from build123d import *

# Parameters (mm, degrees)
EXTRUDE_1_DEPTH          = 64
CUT_EXTRUDE_1_DEPTH      = 850.57468483
CUT_EXTRUDE_1_DEPTH_BACK = 850.57468483
SKETCH_2_R               = 20
SKETCH_4_R               = 140
EXTRUDE_4_DEPTH          = 500
SHELL_6_T                = -5


with BuildPart() as part:
    # 草图1 → 凸台-拉伸1 (new body)
    with BuildSketch(Plane.XY):
        with BuildLine():
            Line((-567.059552989, 207.601354358), (-417.059552989, 207.601354358))
            Line((-417.059552989, 207.601354358), (-417.059552989, 475.601354358))
            Line((-417.059552989, 475.601354358), (-567.059552989, 475.601354358))
            ThreePointArc((-567.059552989, 475.601354358), (-701.059552989, 341.601354358), (-567.059552989, 207.601354358))
        make_face()
    extrude(amount=EXTRUDE_1_DEPTH)

    # 草图2 → 切除-拉伸1 (cut, two sides: drawn at the far end of the back side and taken through both)
    with BuildSketch(Plane.XY.offset(64).offset(-CUT_EXTRUDE_1_DEPTH_BACK)):
        with Locations((-627.059552989, 342.387508152)):
            Circle(SKETCH_2_R)
    extrude(amount=CUT_EXTRUDE_1_DEPTH + CUT_EXTRUDE_1_DEPTH_BACK, mode=Mode.SUBTRACT)

    # 草图4 → 凸台-拉伸4 (add)
    with BuildSketch(Plane(origin=(-417.059552989, 0, 0), x_dir=(0, 0, -1), z_dir=(1, 0, 0))):
        with Locations(Location((-32, 341.601354358, 0), (0, 0, 90))):
            Circle(SKETCH_4_R)
    extrude(amount=EXTRUDE_4_DEPTH)

    # 抽壳6
    shell_6_openings = [part.faces().sort_by_distance(p)[0] for p in [
        (82.940447011, 341.601354358, 32),
    ]]
    offset(amount=SHELL_6_T, openings=shell_6_openings, kind=Kind.INTERSECTION)


solid = part.part
Could you check a few things on this model? Use its own coordinates, in mm. A direction names the side the tool comes from. Give positions to 0.01 mm unless a question says otherwise; leave off trailing zeros. Loops run counter-clockwise (first coordinate to the right, second up) from the corner with the lowest first, then second, coordinate; pieces in that order, holes last. Notation, with made-up numbers: M -17.75,25.5 L -0.75,25.5 A14 ccw -0.75,40.5 Z; hole C 4.25,-5 d1. An arc over 180 degrees is marked long. Answer as a JSON object with one key per item and string values.
Q1. Suppose I cut it at C-C, the plane y = 238. List the corners of the cut face in (x, z) for me, plus the area to 3 significant figures.
Values found:
{"outline": "M -652.05,0 L -417.06,0 L -417.06,-62.16 L 82.94,-62.16 L 82.94,-54.55 L -412.06,-54.55 L -412.06,5 L -643.92,5 L -643.92,59 L -412.06,59 L -412.06,118.55 L 82.94,118.55 L 82.94,126.16 L -417.06,126.16 L -417.06,64 L -652.05,64 Z", "area": "11,000 mm²"}
Q2. If I drill on probe 1 along Y at (x, z) = (-612.5, 34.5); probe 2 along Z at (x, y) = (-591.5, 441); probe 3 along X at (y, z) = (423, -2), over which ranges is the centre line in solid material (lowest first)? Write a range as [from, to].
Values found:
{"probe 1": "y = [215.54, 220.87], [322.06, 328.68], [356.1, 362.71], [462.33, 467.66]", "probe 2": "z = [0, 5], [59, 64]", "probe 3": "x = [-417.06, -412.06]"}
Q3. For P1, Ø1.5, axis at x = -90.5, y = 439.5, coming from the +Z side; P2, Ø12, axis at x = -167, z = 119, coming from the -Y side; P3, Ø4, axis at x = -495, y = 269.5, coming from the -Z side, each with a flat end and sliding along its axis, tell me the tip position at first contact or that it passes through.
Values found:
{"P1": "stops at z = 132.81", "P2": "stops at y = 227.41", "P3": "stops at z = 0"}
Q4. Suppose I cut it at B-B, the plane x = -489. List the corners of the cut face in (y, z) for me, plus the area to 3 significant figures.
Values found:
{"outline": "M 207.6,0 L 475.6,0 L 475.6,64 L 207.6,64 Z; hole M 212.6,5 L 470.6,5 L 470.6,59 L 212.6,59 Z", "area": "3,220 mm²"}
Q5. If we mould it in two halves opening along Y, with no side actions, what happens to faces 1 (the flat face through (-488, 470.601, 32)), 2 (the flat face through (-417.06, 340, 65)), 3 (the cylindrical face through (-701.027, 344.548, 31.552))? For each: pulls with the +Y half, pulls with the -Y half, needs draft (parallel to the pull), parting line crosses it, or undercut.
Values found:
{"face 1": "undercut", "face 2": "needs draft", "face 3": "parting line crosses it"}
Q6. Suppose I cut it at D-D, the plane z = -30.5. List the corners of the cut face in (x, y) for me.
Values found:
{"outline": "M -417.06,216.33 L 82.94,216.33 L 82.94,221.94 L -412.06,221.94 L -412.06,461.26 L 82.94,461.26 L 82.94,466.88 L -417.06,466.88 Z"}
Q7. For faces 4 (the flat face through (-491, 475.601, 32)), 5 (the flat face through (-561, 343, 0)), 6 (the flat face through (-493, 207.601, 32)), 7 (the cylindrical face through (-646.9, 327.18, 31.62)), 8 (the flat face through (-491, 212.601, 32)), which set-ups out of +Z, -Z, +X, -X, +Y, -Y let a thin tool reach every point of the face, with its end or its side?
Values found:
{"face 4": "+Z, -Z, -X, +Y", "face 5": "-Z, -X, +Y, -Y", "face 6": "+Z, -Z, -X, -Y", "face 7": "none", "face 8": "+X"}
Q8. Suppose I cut it at A-A, the plane z = 32. List the corners of the cut face in (x, y) for me.
Values found:
{"outline": "C -627.06,342.39 d50; M -567.06,207.6 L -417.06,207.6 L -417.06,201.6 L 82.94,201.6 L 82.94,206.6 L -412.06,206.6 L -412.06,212.6 L -567.06,212.6 A129 cw -567.06,470.6 L -412.06,470.6 L -412.06,476.6 L 82.94,476.6 L 82.94,481.6 L -417.06,481.6 L -417.06,475.6 L -567.06,475.6 A134 ccw Z; hole C -627.06,342.39 d40"}
